The listing builds one solid part. Answer for the finished solid, in the listing's coordinates (mm). A direction names the side the tool comes from. Give positions to 0.01 mm unless a question says otherwise; leave off trailing zeros. Order: outer loops, then holes, each group sorted by start corner. A loop starts at its lowest first (then second) coordinate and runs counter-clockwise, first axis right, second up. Notation, with made-up numbers: (64.25, -4) - (85.25, -4) arc R23 ccw to (85.25, 17) - close; hole circle Ø6 at (57.25, 73). An arc over 180 degrees is marked (long way). Answer in a Markdown table with one row per item.
from build123d import *

# Parameters (mm, degrees)
EXTRUDE_1_DEPTH          = 4
EXTRUDE_3_DEPTH          = 58
CUT_EXTRUDE_6_DEPTH      = 11.5
CUT_EXTRUDE_4_DEPTH      = 15.7
CUT_EXTRUDE_3_DEPTH      = 7.5
CUT_EXTRUDE_7_DEPTH      = 130.011627383
CUT_EXTRUDE_7_DEPTH_BACK = 130.011627383
SKETCH_11_R              = 2.6
SKETCH_12_R              = 5
CUT_EXTRUDE_8_DEPTH      = 58
SKETCH_16_R              = 5
CUT_EXTRUDE_11_DEPTH     = 13
SKETCH_13_R              = 5
CUT_EXTRUDE_9_DEPTH      = 7
SKETCH_14_R              = 2.6
CUT_EXTRUDE_10_DEPTH     = 4
CHAMFER_1_SIZE           = 0.4
FILLET_1_R               = 1.5
FILLET_2_R               = 2.5


with BuildPart() as part:
    # Эскиз1 → Бобышка-Вытянуть1 (new body)
    with BuildSketch(Plane.XY):
        Polygon((0, 0), (80, 0), (80, 40), (60, 40), (40, 60), (40, 80), (0, 80), align=None)
    extrude(amount=EXTRUDE_1_DEPTH)

    # Эскиз7 → Бобышка-Вытянуть3 (add)
    with BuildSketch(Plane.XY.offset(4)):
        Polygon((64, 24), (64, 0), (20, 0), (20, 20), (0, 20), (0, 80), (40, 80), (40, 24), align=None)
    extrude(amount=EXTRUDE_3_DEPTH)

    # Эскиз9 → Вырез-Вытянуть6 (cut, symmetric)
    with BuildSketch(Plane.XY.offset(28.5)):
        Polygon((20, 80), (40, 80), (40, 24), (38.8, 24), (38.8, 4), (21.2, 4), (21.2, 24), (20, 24), align=None)
    extrude(amount=CUT_EXTRUDE_6_DEPTH, both=True, mode=Mode.SUBTRACT)

    # Эскиз8 → Вырез-Вытянуть4 (cut, symmetric)
    with BuildSketch(Plane.XY.offset(28.5)):
        with BuildLine():
            Line((25, 10), (25, 80))
            Line((25, 80), (35, 80))
            Line((35, 80), (35, 10))
            ThreePointArc((35, 10), (30, 5), (25, 10))
        make_face()
    extrude(amount=CUT_EXTRUDE_4_DEPTH, both=True, mode=Mode.SUBTRACT)

    # Эскиз6 → Вырез-Вытянуть3 (cut, symmetric)
    with BuildSketch(Plane.XY.offset(42.5)):
        with BuildLine():
            Line((41.6, 24), (45, 24))
            Line((45, 24), (45, 18.660254038))
            ThreePointArc((45, 18.660254038), (55, 18.660254038), (60, 10))
            Line((60, 10), (60, 5.6))
            Line((60, 5.6), (64, 5.6))
            Line((64, 5.6), (64, 0))
            Line((64, 0), (40, 0))
            Line((40, 0), (40, 10))
            ThreePointArc((40, 10), (40.408336953, 12.828427125), (41.6, 15.425863987))
            Line((41.6, 15.425863987), (41.6, 24))
        make_face()
    extrude(amount=CUT_EXTRUDE_3_DEPTH, both=True, mode=Mode.SUBTRACT)

    # Эскиз11 → Вырез-Вытянуть7 (cut, two sides: drawn at the far end of the back side and taken through both)
    with BuildSketch(Plane(origin=(0, 0, 0), x_dir=(-1, 0, 0), z_dir=(0, 0, -1)).offset(-CUT_EXTRUDE_7_DEPTH_BACK)):
        with Locations(Location((-10, 10, 0), (0, 0, 180))):
            Circle(SKETCH_11_R)
        with Locations((-30, 30)):
            Circle(SKETCH_11_R)
        with Locations((-30, 50)):
            Circle(SKETCH_11_R)
        with Locations((-30, 70)):
            Circle(SKETCH_11_R)
        with Locations((-10, 30)):
            Circle(SKETCH_11_R)
        with Locations((-10, 50)):
            Circle(SKETCH_11_R)
        with Locations((-10, 70)):
            Circle(SKETCH_11_R)
        with Locations(Location((-50, 10, 0), (0, 0, 180))):
            Circle(SKETCH_11_R)
        with Locations(Location((-50, 30, 0), (0, 0, 180))):
            Circle(SKETCH_11_R)
        with Locations(Location((-70, 10, 0), (0, 0, 180))):
            Circle(SKETCH_11_R)
        with Locations(Location((-70, 30, 0), (0, 0, 180))):
            Circle(SKETCH_11_R)
        with Locations((-30, 10)):
            Circle(SKETCH_11_R)
    extrude(amount=CUT_EXTRUDE_7_DEPTH + CUT_EXTRUDE_7_DEPTH_BACK, mode=Mode.SUBTRACT)

    # Эскиз12 → Вырез-Вытянуть8 (cut)
    with BuildSketch(Plane.XY.offset(62)):
        with Locations((10, 70)):
            Circle(SKETCH_12_R)
        with Locations((10, 50)):
            Circle(SKETCH_12_R)
        with Locations((10, 30)):
            Circle(SKETCH_12_R)
    extrude(amount=-CUT_EXTRUDE_8_DEPTH, mode=Mode.SUBTRACT)

    # Эскиз16 → Вырез-Вытянуть11 (cut)
    with BuildSketch(Plane.XY.offset(17)):
        with Locations((30, 70)):
            Circle(SKETCH_16_R)
        with Locations((30, 50)):
            Circle(SKETCH_16_R)
        with Locations((30, 30)):
            Circle(SKETCH_16_R)
        with Locations((30, 10)):
            Circle(SKETCH_16_R)
    extrude(amount=-CUT_EXTRUDE_11_DEPTH, mode=Mode.SUBTRACT)

    # Эскиз13 → Вырез-Вытянуть9 (cut)
    with BuildSketch(Plane.XY.offset(62)):
        with Locations((50, 10)):
            Circle(SKETCH_13_R)
    extrude(amount=-CUT_EXTRUDE_9_DEPTH, mode=Mode.SUBTRACT)

    # Эскиз14 → Вырез-Вытянуть10 (cut)
    with BuildSketch(Plane.XZ):
        with Locations(Location((30, 28.5, 0), (0, 0, 270))):
            Circle(SKETCH_14_R)
    extrude(amount=-CUT_EXTRUDE_10_DEPTH, mode=Mode.SUBTRACT)

    # Фаска1
    chamfer_1_edges = [part.edges().sort_by_distance(p)[0] for p in [
        (20, 80, 28.5),
        (21.2, 24, 28.5),
        (38.8, 24, 28.5),
        (25, 80, 42.1),
        (35, 80, 42.1),
        (30, 80, 12.8),
        (25, 80, 14.9),
        (35, 80, 14.9),
        (30, 80, 44.2),
    ]]
    chamfer(chamfer_1_edges, length=CHAMFER_1_SIZE)

    # Скругление1
    fillet_1_edges = [part.edges().sort_by_distance(p)[0] for p in [
        (20, 20, 33),
    ]]
    fillet(fillet_1_edges, radius=FILLET_1_R)

    # Скругление2
    # the kernel refuses this fillet: 2.5 mm, written as the material it adds along each edge
    with BuildSketch(Plane(origin=(40, 60, 0), x_dir=(0, 1, 0), z_dir=(0, 0, 1))) as fillet_2_piece_1:
        with BuildLine():
            CenterArc((FILLET_2_R * 0.414213562373, -FILLET_2_R), FILLET_2_R, 90, 45)
            Line((-FILLET_2_R * 0.292893218813, -FILLET_2_R * 0.292893218813), (0, 0))
            Line((0, 0), (FILLET_2_R * 0.414213562373, 0))
        make_face()
    extrude(amount=4)
    with BuildSketch(Plane(origin=(60, 40, 0), x_dir=(1, 0, 0), z_dir=(0, 0, 1))) as fillet_2_piece_2:
        with BuildLine():
            CenterArc((FILLET_2_R * 0.414213562373, FILLET_2_R), FILLET_2_R, 225, 45)
            Line((-FILLET_2_R * 0.292893218813, FILLET_2_R * 0.292893218813), (0, 0))
            Line((0, 0), (FILLET_2_R * 0.414213562373, 0))
        make_face()
    extrude(amount=4)
    with BuildSketch(Plane(origin=(40, 24, 40), x_dir=(1, 0, 0), z_dir=(0, 0, 1))) as fillet_2_piece_3_section:
        with BuildLine():
            CenterArc((FILLET_2_R, FILLET_2_R), FILLET_2_R, 180, 90)
            Line((0, FILLET_2_R), (0, 0))
            Line((0, 0), (FILLET_2_R, 0))
        make_face()
    fillet_2_piece_3 = extrude(amount=22, mode=Mode.PRIVATE)
    fillet_2_piece_3 = split(fillet_2_piece_3, bisect_by=Plane(origin=(41.6, 24.577940424, 45), z_dir=(-1, 0, 0)), keep=Keep.TOP, mode=Mode.PRIVATE)
    add(fillet_2_piece_3)
    with BuildSketch(Plane(origin=(40, 24, 33.75), x_dir=(1, 0, 0), z_dir=(0, 0, 1))) as fillet_2_piece_4_section:
        with BuildLine():
            CenterArc((FILLET_2_R, FILLET_2_R), FILLET_2_R, 180, 90)
            Line((0, FILLET_2_R), (0, 0))
            Line((0, 0), (FILLET_2_R, 0))
        make_face()
    fillet_2_piece_4 = extrude(amount=28.25, mode=Mode.PRIVATE)
    fillet_2_piece_4 = split(fillet_2_piece_4, bisect_by=Plane(origin=(41.823463769, 24.049982966, 50), z_dir=(0, 0, 1)), keep=Keep.TOP, mode=Mode.PRIVATE)
    add(fillet_2_piece_4)
    with BuildSketch(Plane(origin=(40, 24, 4), x_dir=(1, 0, 0), z_dir=(0, 0, 1))) as fillet_2_piece_5:
        with BuildLine():
            CenterArc((FILLET_2_R, FILLET_2_R), FILLET_2_R, 180, 90)
            Line((0, FILLET_2_R), (0, 0))
            Line((0, 0), (FILLET_2_R, 0))
        make_face()
    extrude(amount=13)
    # the kernel refuses this fillet: 2.5 mm, written as the material it takes off along each edge
    with BuildSketch(Plane(origin=(0, 80, 68.25), x_dir=(1, 0, 0), z_dir=(0, 0, -1))) as fillet_2_2_piece_1:
        with BuildLine():
            CenterArc((FILLET_2_R, FILLET_2_R), FILLET_2_R, 180, 90)
            Line((0, FILLET_2_R), (0, 0))
            Line((0, 0), (FILLET_2_R, 0))
        make_face()
    extrude(amount=74.5, mode=Mode.SUBTRACT)
    with BuildSketch(Plane(origin=(40, 80, 68.25), x_dir=(0, -1, 0), z_dir=(0, 0, -1))) as fillet_2_2_piece_2:
        with BuildLine():
            CenterArc((FILLET_2_R, FILLET_2_R), FILLET_2_R, 180, 90)
            Line((0, FILLET_2_R), (0, 0))
            Line((0, 0), (FILLET_2_R, 0))
        make_face()
    extrude(amount=34.5, mode=Mode.SUBTRACT)
    with BuildSketch(Plane(origin=(80, 40, -6.25), x_dir=(-1, 0, 0), z_dir=(0, 0, 1)), Plane(origin=(80, 0, -6.25), x_dir=(0, 1, 0), z_dir=(0, 0, 1))) as fillet_2_2_piece_3:
        with BuildLine():
            CenterArc((FILLET_2_R, FILLET_2_R), FILLET_2_R, 180, 90)
            Line((0, FILLET_2_R), (0, 0))
            Line((0, 0), (FILLET_2_R, 0))
        make_face()
    extrude(amount=16.5, mode=Mode.SUBTRACT)
    with BuildSketch(Plane(origin=(0, 0, -6.25), x_dir=(0, 1, 0), z_dir=(0, 0, 1))) as fillet_2_2_piece_4:
        with BuildLine():
            CenterArc((FILLET_2_R, -FILLET_2_R), FILLET_2_R, 90, 90)
            Line((0, -FILLET_2_R), (0, 0))
            Line((0, 0), (FILLET_2_R, 0))
        make_face()
    extrude(amount=16.5, mode=Mode.SUBTRACT)
    with BuildSketch(Plane(origin=(20, 0, 4), x_dir=(0, 1, 0), z_dir=(0, 0, 1)), Plane(origin=(64, 24, 4), x_dir=(0, -1, 0), z_dir=(0, 0, 1)), Plane(origin=(0, 20, 4), x_dir=(0, 1, 0), z_dir=(0, 0, 1))) as fillet_2_2_piece_5:
        with BuildLine():
            CenterArc((FILLET_2_R, -FILLET_2_R), FILLET_2_R, 90, 90)
            Line((0, -FILLET_2_R), (0, 0))
            Line((0, 0), (FILLET_2_R, 0))
        make_face()
    extrude(amount=64.25, mode=Mode.SUBTRACT)
    with BuildSketch(Plane(origin=(64, 0, 43.75), x_dir=(0, 1, 0), z_dir=(0, 0, 1))) as fillet_2_2_piece_6:
        with BuildLine():
            CenterArc((FILLET_2_R, FILLET_2_R), FILLET_2_R, 180, 90)
            Line((0, FILLET_2_R), (0, 0))
            Line((0, 0), (FILLET_2_R, 0))
        make_face()
    extrude(amount=24.5, mode=Mode.SUBTRACT)
    with BuildSketch(Plane(origin=(40, 80, 23.25), x_dir=(0, -1, 0), z_dir=(0, 0, -1))) as fillet_2_2_piece_7:
        with BuildLine():
            CenterArc((FILLET_2_R, FILLET_2_R), FILLET_2_R, 180, 90)
            Line((0, FILLET_2_R), (0, 0))
            Line((0, 0), (FILLET_2_R, 0))
        make_face()
    extrude(amount=29.5, mode=Mode.SUBTRACT)
    with BuildSketch(Plane(origin=(64, 0, 4), x_dir=(0, 1, 0), z_dir=(0, 0, 1))) as fillet_2_2_piece_8:
        with BuildLine():
            CenterArc((FILLET_2_R, FILLET_2_R), FILLET_2_R, 180, 90)
            Line((0, FILLET_2_R), (0, 0))
            Line((0, 0), (FILLET_2_R, 0))
        make_face()
    extrude(amount=37.25, mode=Mode.SUBTRACT)


with BuildPart() as body_2:
    # Зеркальное отражение1: mirrored copy
    add(part.part.mirror(Plane(origin=(0, 0, 0), x_dir=(0, 0, 1), z_dir=(1, 0, 0))))


solid = body_2.part
Item 1: Find section C-C on x = -50. Write down the section's boundary in (y, z), then the cut area to 3 significant figures.
Answer block:
| item | result |
|---|---|
| outline | (0, 0) - (7.4, 0) - (7.4, 35) - (0, 35) - close; (0, 50) - (7.4, 50) - (7.4, 55) - (5, 55) - (5, 62) - (0, 62) - close; (12.6, 0) - (27.4, 0) - (27.4, 4) - (24, 4) - (24, 62) - (15, 62) - (15, 55) - (12.6, 55) - (12.6, 50) - (20, 50) - (20, 35) - (12.6, 35) - close; (32.6, 0) - (50, 0) - (50, 4) - (32.6, 4) - close |
| area | 993 mm² |
Item 2: Each of these flat-tipped pins is pushed along its axis until it touches: P1, Ø1, axis at x = -45.5, y = 54.5, coming from the +Z side; P2, Ø5, axis at y = 40.5, z = 41, coming from the -X side; P3, Ø21.5, axis at y = 12, z = 30.5, coming from the -X side. Where does it stop, or does it pass through?
Answer block:
| item | result |
|---|---|
| P1 | z = 4 |
| P2 | x = -40 |
| P3 | x = -64 |
Item 3: Find section A-A on z = 28.5. Count the separate pieces of the cut face and the enclosed holes in it, then the cut area to 3 significant figures.
Answer block:
| item | result |
|---|---|
| separate pieces | 2 |
| enclosed holes | 4 |
| area | 1,620 mm² |
Item 4: Determine the mould class of faces 4 (the face through (-30, 40, 12.8)), 5 (the face through (-41, 0, 24)), 6 (the face through (-14.619, 28.085, 33.406)), 7 (the face through (-69, 40, 2)) for opening direction Y: pulls with the +Y half, pulls with the -Y half, needs draft (parallel to the pull), parting line crosses it, or undercut.
Answer block:
| item | result |
|---|---|
| face 4 | needs draft |
| face 5 | pulls with the -Y half |
| face 6 | undercut |
| face 7 | pulls with the +Y half |
Item 5: Which of the six approach directions +Z, -Z, +X, -X, +Y, -Y give full straight-line access (tool end or side, diameter ignored) to faces 1 (the face through (-36, 43, 40)), 2 (the face through (-40, 5, 43)), 3 (the face through (-13, 54, 33))?
Answer block:
| item | result |
|---|---|
| face 1 | +Y |
| face 2 | -Y |
| face 3 | +Z |
Item 6: Consider line 1 (Y direction, x = -10, z = 35); line 2 (Y direction, x = -8, z = 23.5); line 3 (Y direction, x = -10, z = 2). Determine where each line is inside the solid, lowest interval first.
Answer block:
| item | result |
|---|---|
| line 1 | 20 to 25, 35 to 45, 55 to 65, 75 to 80 |
| line 2 | 20 to 25.42, 34.58 to 45.42, 54.58 to 65.42, 74.58 to 80 |
| line 3 | 0 to 7.4, 12.6 to 27.4, 32.6 to 47.4, 52.6 to 67.4, 72.6 to 80 |
